For this review, take the finished solid that the model builds, in its own axes (mm). Round coordinates to 2 decimals unless told otherwise and drop trailing zeros. Write each loop counter-clockwise with the first axis right and the second up, starting at its lowest first coordinate (ties: lowest second). Pieces come first, ordered by that corner, then holes. Notation, with made-up numbers: M 8.5,43 L 50.5,43 A26 ccw 50.5,76 Z; hole C 60.25,60 d9. An arc over 180 degrees is marked long. One line per question, with ' | ' between items.
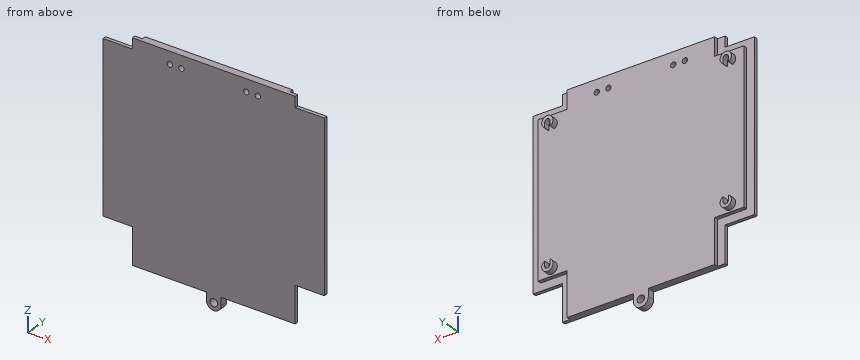
```python
from build123d import *

# Parameters (mm, degrees)
BOSS_EXTRUDE1_DEPTH = 6.35
CUT_EXTRUDE1_DEPTH  = 3.375
SKETCH3_W           = 12.7
SKETCH3_H           = 12.7
BOSS_EXTRUDE2_DEPTH = 6.35
FILLET1_R           = 6.35
SKETCH4_R           = 3.175
CUT_EXTRUDE2_DEPTH  = 255.013969616
SKETCH5_R           = 2.286
CUT_EXTRUDE3_DEPTH  = 12.7
BOSS_EXTRUDE3_DEPTH = 5.08


with BuildPart() as part:
    # Sketch1 → Boss-Extrude1 (new body)
    with BuildSketch(Plane(origin=(0, 0, 0), x_dir=(1, 0, 0), z_dir=(0, 1, 0))):
        Polygon((0, 150.29942), (0, 181.102), (139.192, 181.102), (139.192, 150.29942), (164.084, 150.29942), (164.084, 8.95858), (139.192, 8.95858), (139.192, 0), (0, 0), (0, 8.95858), (-24.892, 8.95858), (-24.892, 150.29942), align=None)
    extrude(amount=BOSS_EXTRUDE1_DEPTH)

    # Sketch2 → Cut-Extrude1 (cut)
    with BuildSketch(Plane(origin=(0, 6.35, 0), x_dir=(1, 0, 0), z_dir=(0, 1, 0))):
        Polygon((132.6420004, 181.102), (132.6420004, 143.7494204), (157.5340004, 143.7494204), (157.5340004, 15.5085796), (132.6420004, 15.5085796), (132.6420004, 0), (139.192, 0), (139.192, 8.95858), (164.084, 8.95858), (164.084, 150.29942), (139.192, 150.29942), (139.192, 181.102), align=None)
        Polygon((0, 181.102), (6.5499996, 181.102), (6.5499996, 143.7494204), (-18.3420004, 143.7494204), (-18.3420004, 15.5085796), (6.5499996, 15.5085796), (6.5499996, 0), (0, 0), (0, 8.95858), (-24.892, 8.95858), (-24.892, 150.29942), (0, 150.29942), align=None)
    extrude(amount=-CUT_EXTRUDE1_DEPTH, mode=Mode.SUBTRACT)

    # Sketch3 → Boss-Extrude2 (add)
    with BuildSketch(Plane(origin=(0, 6.35, 0), x_dir=(1, 0, 0), z_dir=(0, 1, 0))):
        with Locations((69.596, 187.452)):
            Rectangle(SKETCH3_W, SKETCH3_H)
    extrude(amount=-BOSS_EXTRUDE2_DEPTH)

    # Fillet1
    fillet1_edges = [part.edges().sort_by_distance(p)[0] for p in [
        (63.246, 3.175, -193.802),
        (75.946, 3.175, -193.802),
    ]]
    fillet(fillet1_edges, radius=FILLET1_R - 0.0001)  # a hair under: the kernel refuses the full size

    # Sketch4 → Cut-Extrude2 (cut, through all)
    with BuildSketch(Plane(origin=(0, 6.35, 0), x_dir=(1, 0, 0), z_dir=(0, 1, 0))):
        with Locations(Location((69.596, 187.452, 0), (0, 0, 270))):
            Circle(SKETCH4_R)
    extrude(amount=-CUT_EXTRUDE2_DEPTH, mode=Mode.SUBTRACT)

    # Sketch5 → Cut-Extrude3 (cut)
    with BuildSketch(Plane.XZ):
        with Locations(Location((107.188, -10.414, 0), (0, 0, 270))):
            Circle(SKETCH5_R)
        with Locations(Location((97.282, -10.414, 0), (0, 0, 270))):
            Circle(SKETCH5_R)
        with Locations(Location((41.91, -10.414, 0), (0, 0, 270))):
            Circle(SKETCH5_R)
        with Locations(Location((32.004, -10.414, 0), (0, 0, 270))):
            Circle(SKETCH5_R)
    extrude(amount=-CUT_EXTRUDE3_DEPTH, mode=Mode.SUBTRACT)

    # Sketch6 → Boss-Extrude3 (add)
    with BuildSketch(Plane(origin=(0, 6.35, 0), x_dir=(1, 0, 0), z_dir=(0, 1, 0))):
        with BuildLine():
            Line((-4.318, 23.114), (-4.318, 27.364232935))
            ThreePointArc((-4.318, 27.364232935), (-6.604, 18.288), (-8.89, 27.364232935))
            Line((-8.89, 27.364232935), (-8.89, 23.114))
            ThreePointArc((-8.89, 23.114), (-6.604, 20.828), (-4.318, 23.114))
        make_face()
        with BuildLine():
            Line((-8.89, 137.414), (-8.89, 133.163767065))
            ThreePointArc((-8.89, 133.163767065), (-6.604, 142.24), (-4.318, 133.163767065))
            Line((-4.318, 133.163767065), (-4.318, 137.414))
            ThreePointArc((-4.318, 137.414), (-6.604, 139.7), (-8.89, 137.414))
        make_face()
        with BuildLine():
            Line((148.082, 23.114), (148.082, 27.364232935))
            ThreePointArc((148.082, 27.364232935), (145.796, 18.288), (143.51, 27.364232935))
            Line((143.51, 27.364232935), (143.51, 23.114))
            ThreePointArc((143.51, 23.114), (145.796, 20.828), (148.082, 23.114))
        make_face()
        with BuildLine():
            Line((148.082, 137.414), (148.082, 133.163767065))
            ThreePointArc((148.082, 133.163767065), (145.796, 142.24), (143.51, 133.163767065))
            Line((143.51, 133.163767065), (143.51, 137.414))
            ThreePointArc((143.51, 137.414), (145.796, 139.7), (148.082, 137.414))
        make_face()
    extrude(amount=BOSS_EXTRUDE3_DEPTH)


solid = part.part
```
Item 1: Take a section at A-A (x = 41.91). Write out the cut boundary in (y, z).
Results:
outline: M 0,-181.1 L 6.35,-181.1 L 6.35,-12.7 L 0,-12.7 Z; M 0,-8.13 L 6.35,-8.13 L 6.35,0 L 0,0 Z
Item 2: Take a section at B-B (z = -74.5). Write out the cut boundary in (x, y) (3 decimals).
Results:
outline: M -24.892,0 L 164.084,0 L 164.084,2.975 L 157.534,2.975 L 157.534,6.35 L -18.342,6.35 L -18.342,2.975 L -24.892,2.975 Z
Item 3: Insertion check: pin 1 Ø3 at (y, z) = (2.5, -184) entering from +X; pin 2 Ø4.5 at (y, z) = (8.5, -135) entering from -X; pin 3 Ø2.5 at (x, y) = (143, 4.5) entering from -Z. Each pin has a flat end and moves straight along its axis. Give the tip position at first contact, or say it passes through.
Results:
pin 1: x = 75.95 | pin 2: x = -18.34 | pin 3: z = -143.75
Item 4: To check wall thickness, follow line 1 along Z through (x, y) = (42, 3.25); line 2 along Y through (x, z) = (22.5, -72); line 3 along Z through (x, y) = (80, 5.5). State the ranges of each line that lie inside material, in increasing order. Write a range as from..to.
Results:
line 1: -181.1..-12.7, -8.13..0 | line 2: 0..6.35 | line 3: -181.1..0
